Here's how the part is built. I have some questions about the finished solid (model axes, mm). A direction names the side the tool comes from. Coordinates: 2 decimals unless noted, no trailing zeros. Loops run counter-clockwise (first coordinate to the right, second up) from the corner with the lowest first, then second, coordinate; pieces in that order, holes last. Notation, with made-up numbers: (-12, -28) -> (25, -28) arc R35 ccw to (25, 4) -> close; hole circle Ø6 at (68, 2). An arc over 180 degrees is marked (long way). Answer as a JSON object with one key per item and string values. Group by question number.
1) I'm going to push a flat-ended pin straight in: pin 1 (8 mm diameter, centred on x = 64.5, y = 15.5, fed in from +Z). Where does the tip first touch, or does it pass through?
2) If we mould it in two halves opening along X, with no side actions, what happens to faces 3 (the flat face through (-107.107, -9, 100)), 4 (the flat face through (-7, -12, -19.05)), 5 (the flat face through (115.143, -8, 94))? For each: +X half, -X half, draft (parallel to the pull), parting line (faces both ways), or undercut.
3) I want a section at B-B (y = 26). Write out the boundary of the cut face in (x, z).
4) Which directions (+Z, -Z, +X, -X, +Y, -Y) give clear straight access to the entire face, cutting with the end or side of a thin tool? Please do faces 1 (the flat face through (-126.157, -8, 94)), 2 (the flat face through (-7, 94.013, 100)).
5) I want a section at A-A (z = 110). Write out the boundary of the cut face in (x, y).
6) I want a section at C-C (x = -91). Write out the boundary of the cut face in (y, z), then the cut area to 3 significant figures.
7) I need wall thicknesses on probe 1 along X at (y, z) = (-24, 22.5); probe 2 along Y at (x, z) = (17, 50); probe 3 along Z at (x, y) = (-40, -52). Which ranges of each line are inside material? Lowest first, please. Write a range as [from, to].
```python
from build123d import *

# Parameters (mm, degrees)
F1_DEPTH = 203.2
F2_W     = 241.3
F2_H     = 246.338792
F3_DEPTH = 19.05


with BuildPart() as f1:
    # F0 (on Top) → F1 (new body)
    with BuildSketch(Plane.XY):
        Polygon((-107.106747, -109.186523), (-107.106747, -9.808976), (-126.156747, -9.808976), (-126.156747, -133.275315), (115.143253, -133.275315), (115.143253, -7.586523), (96.093253, -7.586523), (96.093253, -109.186523), align=None)
        Polygon((-107.106747, -9.808976), (-107.106747, 94.013477), (-2.590392, 94.013477), (-2.590392, 113.063477), (-126.156747, 113.063477), (-126.156747, -9.808976), align=None)
        Polygon((-2.590392, 113.063477), (-2.590392, 94.013477), (96.093253, 94.013477), (96.093253, -7.586523), (115.143253, -7.586523), (115.143253, 113.063477), align=None)
    extrude(amount=F1_DEPTH)

    # F2 (on face) → F3 (join)
    with BuildSketch(Plane(origin=(0, 0, 0), x_dir=(1, 0, 0), z_dir=(0, 0, -1))):
        with Locations((-5.506747, 10.105919)):
            Rectangle(F2_W, F2_H)
    extrude(amount=F3_DEPTH)


solid = f1.part
```
Determined:
{
 "1": {"pin 1": "z = 0"},
 "2": {"face 3": "undercut", "face 4": "draft", "face 5": "+X half"},
 "3": {"outline": "(-126.16, -19.05) -> (115.14, -19.05) -> (115.14, 203.2) -> (96.09, 203.2) -> (96.09, 0) -> (-107.11, 0) -> (-107.11, 203.2) -> (-126.16, 203.2) -> close"},
 "4": {"face 1": "+Z, -Z, -X, +Y, -Y", "face 2": "+Z"},
 "5": {"outline": "(-126.16, -133.28) -> (115.14, -133.28) -> (115.14, 113.06) -> (-126.16, 113.06) -> close; hole (-107.11, -109.19) -> (96.09, -109.19) -> (96.09, 94.01) -> (-107.11, 94.01) -> close"},
 "6": {"outline": "(-133.28, -19.05) -> (113.06, -19.05) -> (113.06, 203.2) -> (94.01, 203.2) -> (94.01, 0) -> (-109.19, 0) -> (-109.19, 203.2) -> (-133.28, 203.2) -> close", "area": "13,500 mm^2"},
 "7": {"probe 1": "[-126.16, -107.11], [96.09, 115.14]", "probe 2": "[-133.28, -109.19], [94.01, 113.06]", "probe 3": "[-19.05, 0]"}
}
